The model under review builds one solid part; all positions refer to its coordinate system, in mm. A direction names the side the tool comes from. Coordinates: 2 decimals unless noted, no trailing zeros. Loops run counter-clockwise (first coordinate to the right, second up) from the corner with the lowest first, then second, coordinate; pieces in that order, holes last. Notation, with made-up numbers: (18.25, 3) - (45.25, 3) arc R18 ccw to (45.25, 23) - close; hole circle Ø8 at (78.25, 28). An arc over 180 degrees is marked (long way). Use a Markdown table: item, result. Add a question column.
1) Clearance check with flat-ended pins moving along their axes: pin 1 (6.5 mm diameter, centred on x = -15, z = 28, fed in from +Y); pin 2 (5 mm diameter, centred on y = 33, z = 9, fed in from +X); pin 3 (5 mm diameter, centred on y = 26, z = 17.5, fed in from -X); pin 4 (1.8 mm diameter, centred on x = 10, z = 15, fed in from -Y). State where each tip first meets the part, or that it passes through.
2) Add section B-B, the plane y = 25. Give the boundary of the cut face in (x, z), and give its area (3 significant figures).
3) For faces 1 (the flat face through (-32.5, -28, 20)), 2 (the flat face through (32.5, 27, 20)), 3 (the flat face through (0, -22.5, 25)), list the 3-axis set-ups (+Z, -Z, +X, -X, +Y, -Y) from which the entire face can be reached by the end or side of a thin tool; tool diameter is ignored.
4) The part is to be moulded in two halves that separate along X. For faces 4 (the cylindrical face through (-10.9, -27.4, 33.8)), 5 (the flat face through (0, 22.5, 25)), 6 (the flat face through (-32.5, 27, 20)), say which applies: pulls with the +X half, pulls with the -X half, needs draft (parallel to the pull), parting line crosses it, or undercut.
5) Add section C-C, the plane x = 10. Give the boundary of the cut face in (y, z), and give its area (3 significant figures).
6) To check wall thickness, follow L1, parallel to X at y = 28.5, z = 28; L2, parallel to Z at x = -9, y = 27.5; L3, parallel to X at y = -27.5, z = 15. State the ranges of each line that lie inside material, in increasing order. Write a range as [from, to].
7) Add section D-D, the plane x = -28. Give the boundary of the cut face in (y, z), and give its area (3 significant figures).
8) Add section A-A, the plane z = 28. Give the boundary of the cut face in (x, y).
```python
from build123d import *

# Parameters (mm, degrees)
SKETCH_1_R                    = 50
EXTRUDE_1_DEPTH               = 10
HOLE_WIZARD_M10_1_D           = 8.5
HOLE_WIZARD_M10_1_CSINK_D     = 10.05
HOLE_WIZARD_M10_1_CSINK_ANGLE = 90
SKETCH_9_W                    = 65
SKETCH_9_H                    = 10
EXTRUDE_3_DEPTH               = 30
FILLET_2_R                    = 10
SKETCH_14_R                   = 2.5
SKETCH_14_R_2                 = 1.5
CUT_EXTRUDE_3_DEPTH           = 105.432992871


with BuildPart() as part:
    # 草图1 → 凸台-拉伸1 (new body)
    with BuildSketch(Plane.XY):
        Circle(SKETCH_1_R)
    extrude(amount=EXTRUDE_1_DEPTH)

    # M10 螺纹孔1 (through all)
    with Locations(Plane.XY.offset(10)):
        with Locations((-20.426671729, 0)):
            hole_wizard_m10_1 = CounterSinkHole(HOLE_WIZARD_M10_1_D / 2, HOLE_WIZARD_M10_1_CSINK_D / 2, counter_sink_angle=HOLE_WIZARD_M10_1_CSINK_ANGLE)

    # 镜向2: M10 螺纹孔1 across plane
    add(hole_wizard_m10_1.mirror(Plane(origin=(0, 0, 0), x_dir=(0, 0, 1), z_dir=(1, 0, 0))), mode=Mode.SUBTRACT)

    # 草图9 → 凸台-拉伸3 (add)
    with BuildSketch(Plane.XY.offset(10)):
        with Locations((0, 27.5)):
            Rectangle(SKETCH_9_W, SKETCH_9_H)
        with Locations((0, -27.5)):
            Rectangle(SKETCH_9_W, SKETCH_9_H)
    extrude(amount=EXTRUDE_3_DEPTH)

    # 圆角2
    fillet_2_edges = [part.edges().sort_by_distance(p)[0] for p in [
        (32.5, -27.5, 40),
        (-32.5, -27.5, 40),
        (-32.5, 27.5, 40),
        (32.5, 27.5, 40),
    ]]
    fillet(fillet_2_edges, radius=FILLET_2_R)

    # 草图14 → 切除-拉伸3 (cut, through all)
    with BuildSketch(Plane(origin=(0, 32.5, 0), x_dir=(1, 0, 0), z_dir=(0, 1, 0))):
        with Locations(Location((-15, -28, 0), (0, 0, 270))):
            Circle(SKETCH_14_R)
        with Locations(Location((10, -15, 0), (0, 0, 270))):
            Circle(SKETCH_14_R_2)
        with Locations(Location((15, -28, 0), (0, 0, 270))):
            Circle(SKETCH_14_R)
        with Locations(Location((10, -35, 0), (0, 0, 270))):
            Circle(SKETCH_14_R_2)
        with Locations(Location((-10, -15, 0), (0, 0, 270))):
            Circle(SKETCH_14_R_2)
        with Locations(Location((-10, -35, 0), (0, 0, 270))):
            Circle(SKETCH_14_R_2)
    extrude(amount=-CUT_EXTRUDE_3_DEPTH, mode=Mode.SUBTRACT)


solid = part.part
```
From the geometry:
| question | item | result |
|---|---|---|
| 1 | pin 1 | stops at y = 32.5 |
| 1 | pin 2 | stops at x = 39.62 |
| 1 | pin 3 | stops at x = -32.5 |
| 1 | pin 4 | passes through |
| 2 | outline | (-43.3, 0) - (43.3, 0) - (43.3, 10) - (32.5, 10) - (32.5, 30) arc R10 ccw to (22.5, 40) - (-22.5, 40) arc R10 ccw to (-32.5, 30) - (-32.5, 10) - (-43.3, 10) - close; hole circle Ø5 at (-15, 28); hole circle Ø3 at (-10, 15); hole circle Ø3 at (-10, 35); hole circle Ø3 at (10, 15); hole circle Ø3 at (10, 35); hole circle Ø5 at (15, 28) |
| 2 | area | 2,710 mm^2 |
| 3 | face 1 | +Z, -X, +Y, -Y |
| 3 | face 2 | +Z, +X, +Y, -Y |
| 3 | face 3 | +Z, +X, -X |
| 4 | face 4 | undercut |
| 4 | face 5 | needs draft |
| 4 | face 6 | pulls with the -X half |
| 5 | outline | (-48.99, 0) - (48.99, 0) - (48.99, 10) - (32.5, 10) - (32.5, 13.5) - (22.5, 13.5) - (22.5, 10) - (-22.5, 10) - (-22.5, 13.5) - (-32.5, 13.5) - (-32.5, 10) - (-48.99, 10) - close; (-32.5, 16.5) - (-22.5, 16.5) - (-22.5, 33.5) - (-32.5, 33.5) - close; (-32.5, 36.5) - (-22.5, 36.5) - (-22.5, 40) - (-32.5, 40) - close; (22.5, 16.5) - (32.5, 16.5) - (32.5, 33.5) - (22.5, 33.5) - close; (22.5, 36.5) - (32.5, 36.5) - (32.5, 40) - (22.5, 40) - close |
| 5 | area | 1,460 mm^2 |
| 6 | L1 | x = [-32.5, -17.5], [-12.5, 12.5], [17.5, 32.5] |
| 6 | L2 | z = [0, 13.88], [16.12, 33.88], [36.12, 40] |
| 6 | L3 | x = [-32.5, -11.5], [-8.5, 8.5], [11.5, 32.5] |
| 7 | outline | (-41.42, 0) - (41.42, 0) - (41.42, 10) - (32.5, 10) - (32.5, 38.35) - (22.5, 38.35) - (22.5, 10) - (-22.5, 10) - (-22.5, 38.35) - (-32.5, 38.35) - (-32.5, 10) - (-41.42, 10) - close |
| 7 | area | 1,400 mm^2 |
| 8 | outline | (-32.5, -32.5) - (-17.5, -32.5) - (-17.5, -22.5) - (-32.5, -22.5) - close; (-32.5, 22.5) - (-17.5, 22.5) - (-17.5, 32.5) - (-32.5, 32.5) - close; (-12.5, -32.5) - (12.5, -32.5) - (12.5, -22.5) - (-12.5, -22.5) - close; (-12.5, 22.5) - (12.5, 22.5) - (12.5, 32.5) - (-12.5, 32.5) - close; (17.5, -32.5) - (32.5, -32.5) - (32.5, -22.5) - (17.5, -22.5) - close; (17.5, 22.5) - (32.5, 22.5) - (32.5, 32.5) - (17.5, 32.5) - close |
